Autodesk Fusion 360 part; units mm, degrees
sketch "スケッチ1" plane through (0, 0, 0) normal (0, 1, 0) x (1, 0, 0)
  circle A0 centre (0, 0) radius 25
  dimension "d1" = 50
extrude "押し出し1" add sketch "スケッチ1" along normal blind 30
sketch "スケッチ2" plane through (0, 0, 0) normal (0, -1, 0) x (1, 0, 0)
  circle A0 centre (0, 0) radius 25
  circle A1 centre (0, 0) radius 3
  line L0 (0, 1.05) -> (-0.9093, 0.525)
  line L1 (-0.9093, 0.525) -> (-0.9093, -0.525)
  line L2 (-0.9093, -0.525) -> (0, -1.05)
  line L3 (0, -1.05) -> (0.9093, -0.525)
  line L4 (0.9093, -0.525) -> (0.9093, 0.525)
  line L5 (0.9093, 0.525) -> (0, 1.05)
  dimension "d4" = 6
  dimension "d5" = 2.1
extrude "押し出し2" add sketch "スケッチ2" along normal blind 1 contours A1
extrude "押し出し3" cut 1 faces at (0, 0, 0.35) along direction (0, 1, 0) blind 4
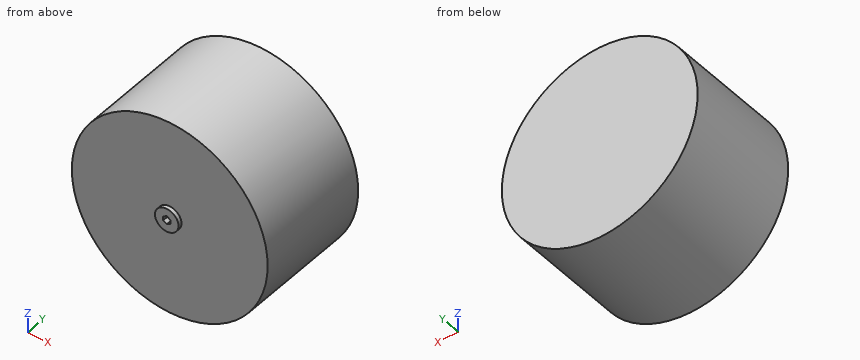
Could you check a few things on this model? Use its own coordinates, in mm. Coordinates: 2 decimals unless noted, no trailing zeros. Loops run counter-clockwise (first coordinate to the right, second up) from the corner with the lowest first, then second, coordinate; pieces in that order, holes last. Notation, with made-up numbers: M 84.25,20 L 140.25,20 A23 ccw 140.25,28 Z; hole C -36.75,-3 d10. An arc over 180 degrees is marked long. Put each result on its own line as item: value. Start each with the question number.
(1) Suppose I cut it at C-C on z = 7. Please give me the cut outline in (x, y).
(2) I need wall thicknesses on line 1 (Y direction, x = -15, z = -10); line 2 (X direction, y = 28, z = 3); line 3 (Z direction, x = 8.5, y = 5.5). Which ranges of each line are inside material? Lowest first, please. Write a range as from..to.
(3) Suppose I cut it at A-A on x = -20. Please give me the cut outline in (y, z), then the cut area to 3 significant figures.
(4) Suppose I cut it at B-B on y = 23. Please give me the cut outline in (x, z).
(5) Will these pins go through, and if not, where does the flat tip stop? P1, Ø1, axis at x = -11.5, z = 3.5, coming from the -Y side; P2, Ø12, axis at y = 14, z = -6.5, coming from the -X side (3 decimals); P3, Ø2, axis at x = 0, z = -0.5, coming from the -Y side; P4, Ø8, axis at y = 7, z = 15, coming from the -X side.
Solutions:
1. outline: M -24,0 L 24,0 L 24,30 L -24,30 Z
2. line 1: y = 0..30
2. line 2: x = -24.82..24.82
2. line 3: z = -23.51..23.51
3. outline: M 0,-15 L 30,-15 L 30,15 L 0,15 Z
3. area: 900 mm2
4. outline: C 0,0 d50
5. P1: stops at y = 0
5. P2: stops at x = -24.995
5. P3: stops at y = -1
5. P4: stops at x = -22.45
